Answer from the drawing. Dimensions are ordinates in mm from the lowest x, y and z of the part. A direction names the side the tool comes from. Coordinates: 2 decimals unless noted, no trailing zeros. Write each loop counter-clockwise with the first axis right and the second up, starting at its lowest first coordinate (ties: lowest second). Pieces come first, ordered by that corner, then holes. Notation, with made-up numbers: (-17, 8.5) -> (25, 8.5) arc R24 cw to (25, 22.5) -> close; hole circle Ø8 at (-37, 20.25). An arc over 180 degrees is marked (long way). One line per item, written item: value. Start each with the question number.
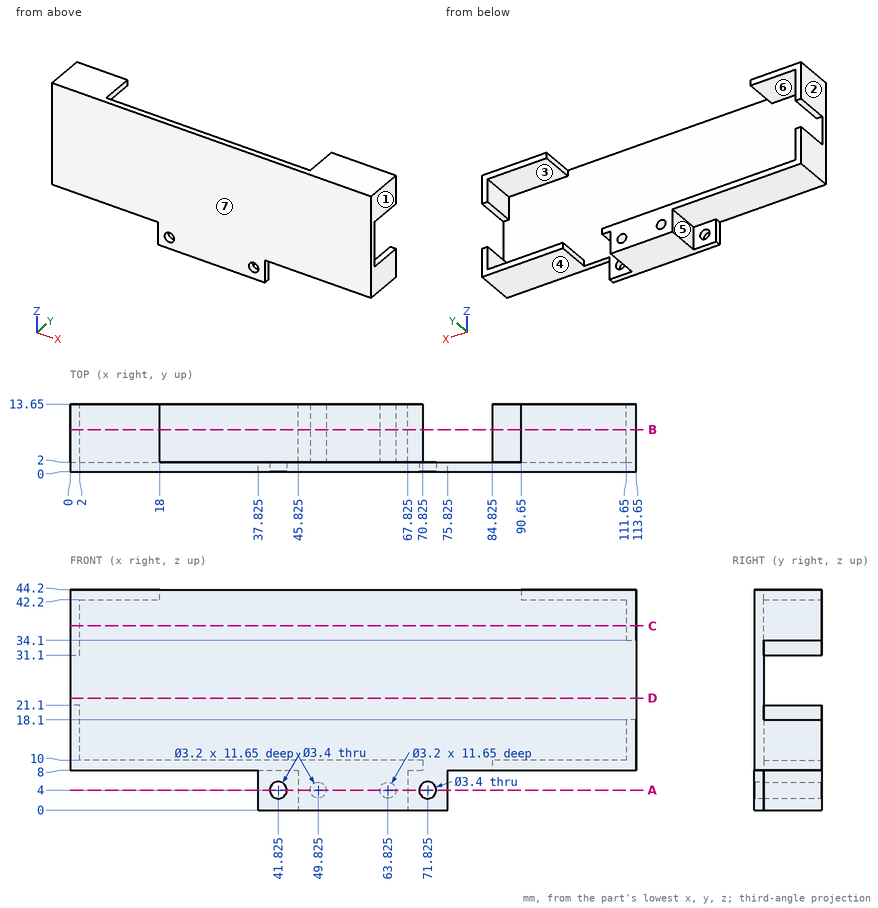
1. A cutting plane is placed at C-C on z = 37. Give the vertices of the cut face in (x, y).
2. Given pin 1 (7 mm diameter, centred on x = 94, y = 9, fed in from -Z); pin 2 (2 mm diameter, centred on x = 71, z = 30.5, fed in from -Y); pin 3 (2.5 mm diameter, centred on y = 5, z = 3, fed in from -X) (3 decimals); pin 4 (6 mm diameter, centred on x = 46.5, y = 10.5, fed in from +Z), each flat-ended and moving along its own axis, determine where each tip first touches the part or whether it passes through.
3. A tool of negligible diameter and unlimited length cuts with its end or side. For the marked faces 4, 5, 6 and 7, from which of +Z, -Z, +X, -X, +Y, -Y can it reach the whole face along a straight path? Write none if from no direction.
4. A cutting plane is placed at D-D on z = 22.5. Give the vertices of the cut face in (x, y).
5. A cutting plane is placed at A-A on z = 4. Give the vertices of the cut face in (x, y) (3 decimals), then the cut area to 3 significant figures.
6. For a pull along X with two mould halves and no side action, classify the marked faces 1, 2 and 3 as +X half, -X half, draft (parallel to the pull), parting line (faces both ways), or undercut.
7. Find the intervals of material crossed by probe 1 along X at (y, z) = (0.75, 4) (3 decimals); probe 2 along X at (y, z) = (5.5, 4) (3 decimals); probe 3 along Z at (x, y) = (93, 11.75), in increasing order. Write a range as from..to.
8. A cutting plane is placed at B-B on y = 8.5. Count the separate pieces of the cut face and the enclosed holes in it, then the cut area to 3 significant figures.
Derived:
1. outline: (0, 0) -> (113.65, 0) -> (113.65, 13.65) -> (111.65, 13.65) -> (111.65, 2) -> (2, 2) -> (2, 13.65) -> (0, 13.65) -> close
2. pin 1: stops at z = 8
2. pin 2: stops at y = 0
2. pin 3: stops at x = 45.825
2. pin 4: stops at z = 10
3. face 4: -Z, +X, +Y, -Y
3. face 5: -Z, -X, +Y
3. face 6: +Y
3. face 7: +Z, -Z, +X, -X, -Y
4. outline: (0, 0) -> (113.65, 0) -> (113.65, 2) -> (0, 2) -> close
5. outline: (37.825, 0) -> (40.125, 0) -> (40.125, 2) -> (37.825, 2) -> close; (43.525, 0) -> (70.125, 0) -> (70.125, 2) -> (67.825, 2) -> (67.825, 13.65) -> (65.425, 13.65) -> (65.425, 2) -> (62.225, 2) -> (62.225, 13.65) -> (51.425, 13.65) -> (51.425, 2) -> (48.225, 2) -> (48.225, 13.65) -> (45.825, 13.65) -> (45.825, 2) -> (43.525, 2) -> close; (73.525, 0) -> (75.825, 0) -> (75.825, 2) -> (73.525, 2) -> close
5. area: 244 mm2
6. face 1: +X half
6. face 2: -X half
6. face 3: undercut
7. probe 1: x = 37.825..40.125, 43.525..70.125, 73.525..75.825
7. probe 2: x = 45.825..48.225, 51.425..62.225, 65.425..67.825
7. probe 3: z = 8..10, 42.2..44.2
8. separate pieces: 4
8. enclosed holes: 2
8. area: 518 mm2
